Geometry check sheet. Reference: drawing and pictorial views, mm from the part's lowest x, y, z. A direction names the side the tool comes from. Give positions to 0.01 mm unless a question says otherwise; leave off trailing zeros. Loops run counter-clockwise (first coordinate to the right, second up) from the corner with the lowest first, then second, coordinate; pieces in that order, holes last. Notation, with made-up numbers: (33.5, 22) -> (67.5, 22) arc R16 ccw to (67.5, 44) -> close; hole circle Ø8 at (78, -10.5). An arc over 180 degrees is marked (long way). Write item = value, one per line. Start each with the question number.
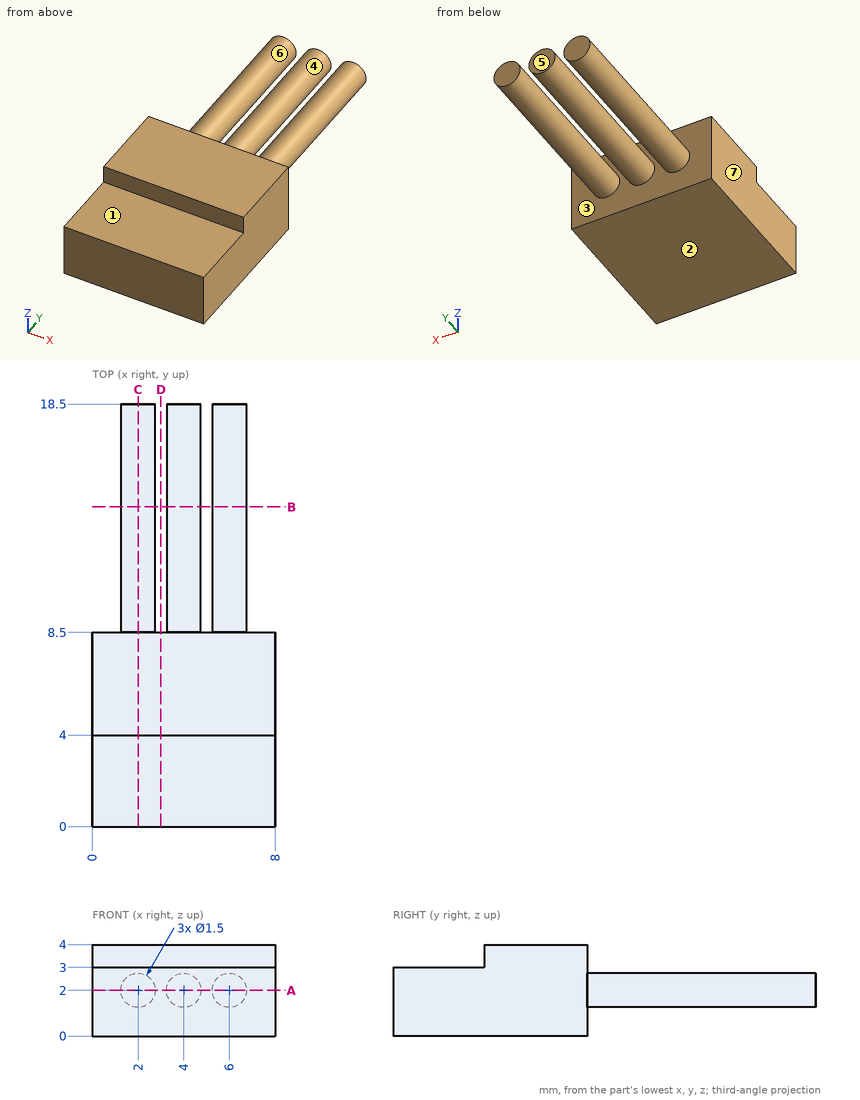
1) Draft check along X on the marked faces 4, 5, 6 and 7. Enter one of: released by +X, released by -X, zero draft, split by the parting line, or undercut.
2) Section check C-C (x = 2). Enter the section's corners in (y, z), plus the area to 3 significant figures.
3) Section check B-B (y = 14). Enter the section's corners in (x, z).
4) Section check D-D (x = 3). Enter the section's corners in (y, z), plus the area to 3 significant figures.
5) Depth check by flat-ended pin: pin 1 Ø1.5 at (y, z) = (15, 1) entering from -X; pin 2 Ø1 at (x, y) = (4, 10) entering from +Z; pin 3 Ø2 at (x, y) = (5, 1) entering from +Z. Enter the tip coordinate at first touch or a pass-through.
6) Thickness scan on line 1 (Y direction, x = 3.75, z = 2.85); line 2 (Y direction, x = 3, z = 3.3); line 3 (Z direction, x = 2, y = 14.25). Record the ranges inside material, lowest first.
7) Tool access check on the marked faces 1, 2 and 3. Record the directions out of +Z, -Z, +X, -X, +Y, -Y that give a thin tool (end or side, any length) a straight path to the whole face; none if there is none.
8) Section check A-A (z = 2). Enter the section's corners in (x, y).
Check result:
q1.face_4 = undercut
q1.face_5 = zero draft
q1.face_6 = undercut
q1.face_7 = released by -X
q2.outline = (0, 0) -> (8.5, 0) -> (8.5, 1.25) -> (18.5, 1.25) -> (18.5, 2.75) -> (8.5, 2.75) -> (8.5, 4) -> (4, 4) -> (4, 3) -> (0, 3) -> close
q2.area = 45.0 mm2
q3.outline = circle Ø1.5 at (2, 2); circle Ø1.5 at (4, 2); circle Ø1.5 at (6, 2)
q4.outline = (0, 0) -> (8.5, 0) -> (8.5, 4) -> (4, 4) -> (4, 3) -> (0, 3) -> close
q4.area = 30.0 mm2
q5.pin_1 = 1.29
q5.pin_2 = 2.75
q5.pin_3 = 3
q6.line_1 = 0 to 8.5
q6.line_2 = 4 to 8.5
q6.line_3 = 1.25 to 2.75
q7.face_1 = +Z, +X, -X, -Y
q7.face_2 = -Z, +X, -X, +Y, -Y
q7.face_3 = +Y
q8.outline = (0, 0) -> (8, 0) -> (8, 8.5) -> (6.75, 8.5) -> (6.75, 18.5) -> (5.25, 18.5) -> (5.25, 8.5) -> (4.75, 8.5) -> (4.75, 18.5) -> (3.25, 18.5) -> (3.25, 8.5) -> (2.75, 8.5) -> (2.75, 18.5) -> (1.25, 18.5) -> (1.25, 8.5) -> (0, 8.5) -> close
